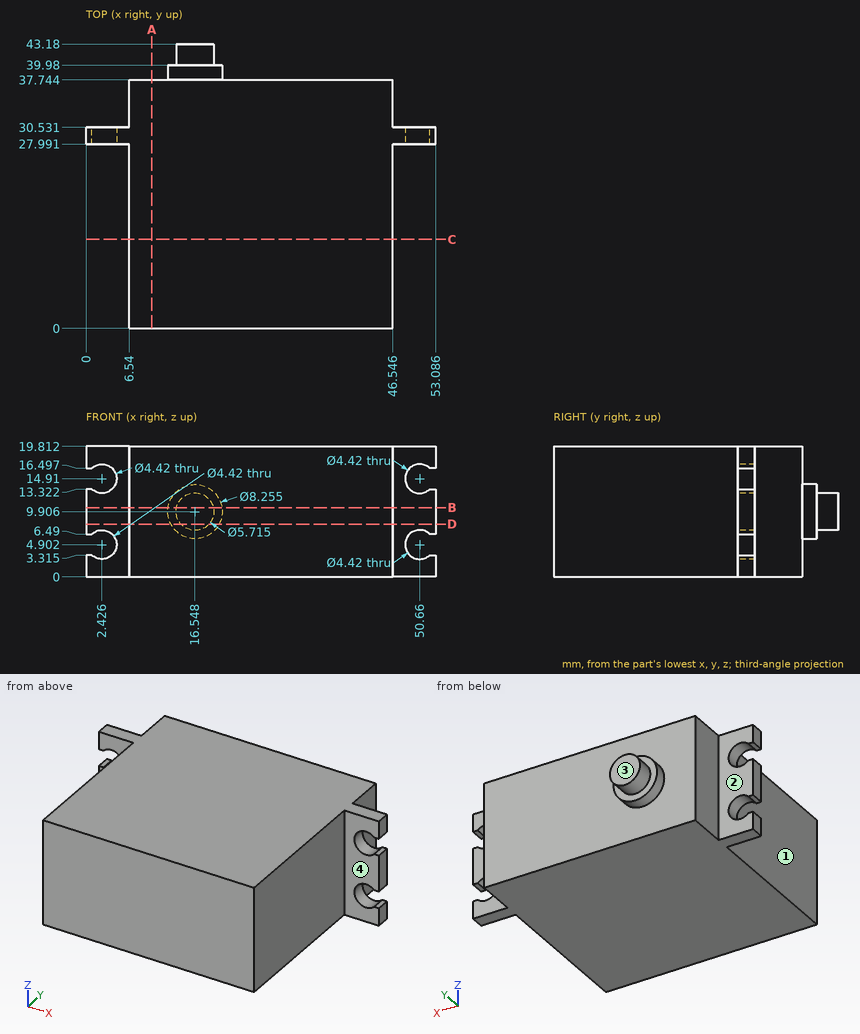
Geometry check sheet. Reference: drawing and pictorial views, mm from the part's lowest x, y, z. A direction names the side the tool comes from. Round coordinates to 2 decimals unless told otherwise and drop trailing zeros. Order: outer loops, then holes, each group sorted by start corner. A loop starts at its lowest first (then second) coordinate and runs counter-clockwise, first axis right, second up.
Q1. Depth check by flat-ended pin: P1, Ø1, axis at x = 52.5, y = 29, coming from the -Z side; P2, Ø5, axis at y = 35, z = 4, coming from the -X side; P3, Ø6, axis at y = 35.5, z = 15, coming from the +X side (1 decimal); P4, Ø2, axis at x = 1.5, z = 8, coming from the -Y side. Enter the tip coordinate at first touch or a pass-through.
Filled sheet:
P1: stops at z = 0
P2: stops at x = 6.54
P3: stops at x = 46.5
P4: stops at y = 27.99
Q2. Set-up check for the marked faces 1, 2, 3 and 4: record each of +Z, -Z, +X, -X, +Y, -Y from which the full face is reachable in a straight line by a thin tool's end or side.
Filled sheet:
face 1: +Z, -Z, -X, -Y
face 2: +Z, -Z, -X, +Y
face 3: +Z, -Z, +X, -X, +Y
face 4: +Z, -Z, +X, -Y
Q3. Cross-section at A-A, the plane x = 10. Enter the section's corners in (y, z) (1 decimal).
Filled sheet:
outline: (0, 0) - (37.7, 0) - (37.7, 19.8) - (0, 19.8) - close
Q4. Cross-section at B-B, the plane z = 10.5. Enter the section's corners in (x, y) (1 decimal), plus the area to 3 significant figures.
Filled sheet:
outline: (0, 28) - (6.5, 28) - (6.5, 0) - (46.5, 0) - (46.5, 28) - (53.1, 28) - (53.1, 30.5) - (46.5, 30.5) - (46.5, 37.7) - (20.6, 37.7) - (20.6, 40) - (19.3, 40) - (19.3, 43.2) - (13.8, 43.2) - (13.8, 40) - (12.5, 40) - (12.5, 37.7) - (6.5, 37.7) - (6.5, 30.5) - (0, 30.5) - close
area: 1,580 mm2
Q5. Cross-section at D-D, the plane z = 8. Enter the section's corners in (x, y) (1 decimal), plus the area to 3 significant figures.
Filled sheet:
outline: (0, 28) - (6.5, 28) - (6.5, 0) - (46.5, 0) - (46.5, 28) - (53.1, 28) - (53.1, 30.5) - (46.5, 30.5) - (46.5, 37.7) - (20.2, 37.7) - (20.2, 40) - (18.7, 40) - (18.7, 43.2) - (14.4, 43.2) - (14.4, 40) - (12.9, 40) - (12.9, 37.7) - (6.5, 37.7) - (6.5, 30.5) - (0, 30.5) - close
area: 1,570 mm2
Q6. Scan lines: L1, parallel to X at y = 8.5, z = 17 (1 decimal); L2, parallel to Y at x = 30, z = 11 (1 decimal); L3, parallel to Y at x = 4, z = 7.5. Record each from-to range of solid material in increasing order.
Filled sheet:
L1: x = 6.5 to 46.5
L2: y = 0 to 37.7
L3: y = 27.99 to 30.53
Q7. Cross-section at C-C, the plane y = 13.5. Enter the section's corners in (x, z) (1 decimal).
Filled sheet:
outline: (6.5, 0) - (46.5, 0) - (46.5, 19.8) - (6.5, 19.8) - close
